from build123d import *

# Parameters (mm, degrees)
F1_DEPTH = 457.2


with BuildPart() as f1:
    # F0 (on Front) → F1 (new body)
    with BuildSketch(Plane.XZ):
        with BuildLine():
            Line((203.835, 0), (-203.835, 0))
            ThreePointArc((-203.835, 0), (-207.427102, -1.487898), (-208.915, -5.08))
            Line((-208.915, -5.08), (-208.915, -25.4))
            Line((-208.915, -25.4), (-206.629, -25.4))
            Line((-206.629, -25.4), (-206.629, -4.826))
            ThreePointArc((-206.629, -4.826), (-205.885051, -3.029949), (-204.089, -2.286))
            Line((-204.089, -2.286), (204.089, -2.286))
            ThreePointArc((204.089, -2.286), (205.885051, -3.029949), (206.629, -4.826))
            Line((206.629, -4.826), (206.629, -25.4))
            Line((206.629, -25.4), (208.915, -25.4))
            Line((208.915, -25.4), (208.915, -5.08))
            ThreePointArc((208.915, -5.08), (207.427102, -1.487898), (203.835, 0))
        make_face()
    extrude(amount=-F1_DEPTH)


solid = f1.part
Build history of the part. All positions in model axes, mm. A direction names the side the tool comes from. Coordinates: 2 decimals unless noted, no trailing zeros. Write each loop counter-clockwise with the first axis right and the second up, starting at its lowest first coordinate (ties: lowest second). Pieces come first, ordered by that corner, then holes.
(1) Drill centre lines: line 1 (X direction, y = 342, z = -18.75) (3 decimals); line 2 (Z direction, x = 191.5, y = 265); line 3 (X direction, y = 131.5, z = -2.75). Where is each one in solid material? Low to high.
(2) Cut at C-C on x = 57. List the corners of the cut face in (y, z), and give its area (3 significant figures).
(3) 3-axis set-ups, long thin cutter, end or side, ignore diameter. For faces 1 (the flat face through (206.629, 225, -15)), 2 (the flat face through (3, 225, 0)): which of +Z, -Z, +X, -X, +Y, -Y reach the whole face in a straight line?
(4) Cut at A-A on z = -16.75. List the corners of the cut face in (x, y) (3 decimals).
(5) Pin check, flat tip, straight feed: pin 1 Ø3 at (x, y) = (154.5, 224) entering from -Z. Stop position of the tip, or through.
(6) Mould opens along X. For faces 3 (the flat face through (-206.629, 225, -15)), 4 (the flat face through (-1, 0, -0.4)), 5 (the flat face through (-208.915, 225, -15)) say: pulls with the +X half, pulls with the -X half, needs draft (parallel to the pull), parting line crosses it, or undercut.
(7) Cut at B-B on y = 355. List the corners of the cut face in (x, z) (3 decimals).
Working result:
1. line 1: x = -208.915 to -206.629, 206.629 to 208.915
1. line 2: z = -2.29 to 0
1. line 3: x = -208.35 to -205.55, 205.55 to 208.35
2. outline: (0, -2.29) - (457.2, -2.29) - (457.2, 0) - (0, 0) - close
2. area: 1,050 mm2
3. face 1: -Z, +Y, -Y
3. face 2: +Z, +X, -X, +Y, -Y
4. outline: (-208.915, 0) - (-206.629, 0) - (-206.629, 457.2) - (-208.915, 457.2) - close; (206.629, 0) - (208.915, 0) - (208.915, 457.2) - (206.629, 457.2) - close
5. pin 1: stops at z = -2.29
6. face 3: undercut
6. face 4: needs draft
6. face 5: pulls with the -X half
7. outline: (-208.915, -25.4) - (-206.629, -25.4) - (-206.629, -4.826) arc R2.54 cw to (-204.089, -2.286) - (204.089, -2.286) arc R2.54 cw to (206.629, -4.826) - (206.629, -25.4) - (208.915, -25.4) - (208.915, -5.08) arc R5.08 ccw to (203.835, 0) - (-203.835, 0) arc R5.08 ccw to (-208.915, -5.08) - close
